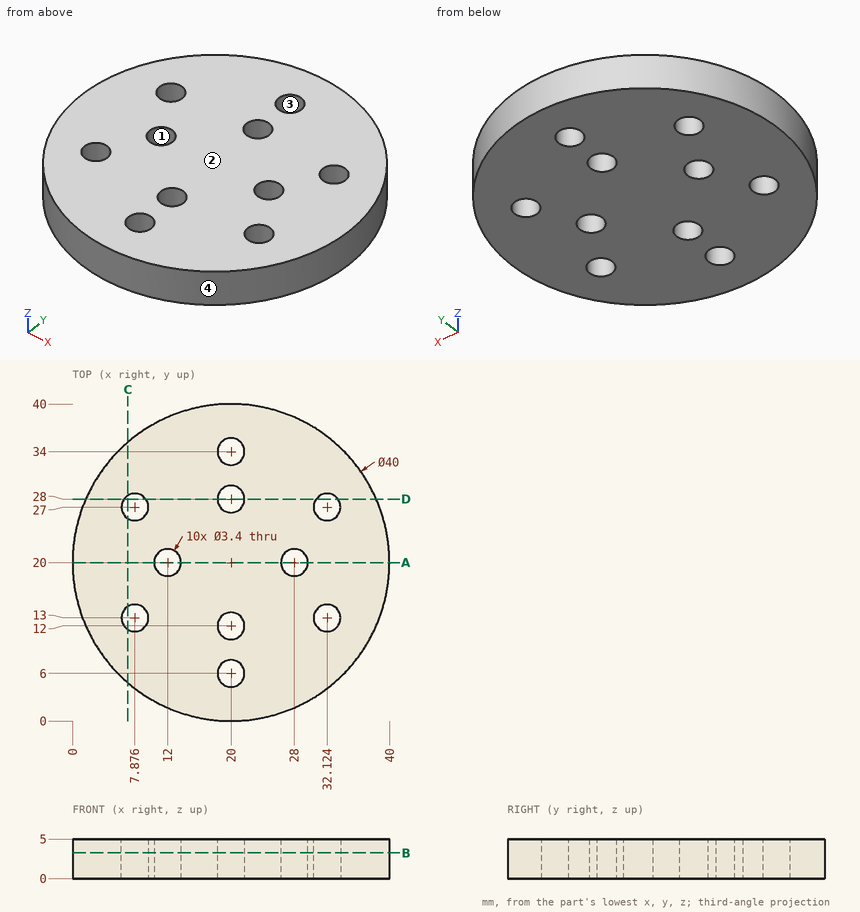
Here's the drawing with two shaded views (mm, measured from the low corner). I have some questions. Give positions to 0.01 mm unless a question says otherwise; leave off trailing zeros. Loops run counter-clockwise (first coordinate to the right, second up) from the corner with the lowest first, then second, coordinate; pieces in that order, holes last. Notation, with made-up numbers: M 1,-22 L 32,-22 A25 cw 32,8 Z; hole C 36,8 d1. An arc over 180 degrees is marked long. One line per item, written item: value.
(1) I need wall thicknesses on line 1 (Y direction, x = 20, z = 2.6); line 2 (X direction, y = 26, z = 1.35); line 3 (Y direction, x = 32, z = 2.95) (1 decimal). Which ranges of each line are inside material? Lowest first, please.
Returned:
line 1: 0 to 4.3, 7.7 to 10.3, 13.7 to 26.3, 29.7 to 32.3, 35.7 to 40
line 2: 0.92 to 6.5, 9.25 to 30.75, 33.5 to 39.08
line 3: 4 to 11.3, 14.7 to 25.3, 28.7 to 36
(2) Suppose I cut it at A-A on y = 20. List the corners of the cut face in (x, z) for me.
Returned:
outline: M 0,0 L 10.3,0 L 10.3,5 L 0,5 Z; M 13.7,0 L 26.3,0 L 26.3,5 L 13.7,5 Z; M 29.7,0 L 40,0 L 40,5 L 29.7,5 Z
(3) We'd pull the mould along X, two halves only. Please class the marked faces 1, 2, 3 and 4: released by +X, released by -X, zero draft, split by the parting line, or undercut.
Returned:
face 1: undercut
face 2: zero draft
face 3: undercut
face 4: split by the parting line
(4) Suppose I cut it at D-D on y = 28. List the corners of the cut face in (x, z) for me.
Returned:
outline: M 1.67,0 L 6.5,0 L 6.5,5 L 1.67,5 Z; M 9.25,0 L 18.3,0 L 18.3,5 L 9.25,5 Z; M 21.7,0 L 30.75,0 L 30.75,5 L 21.7,5 Z; M 33.5,0 L 38.33,0 L 38.33,5 L 33.5,5 Z
(5) Will these pins go through, and if not, where does the flat tip stop? pin 1 (12 mm diameter, centred on x = 23, y = 28.5, fed in from -Z); pin 2 (1 mm diameter, centred on y = 15.5, z = 1.5, fed in from +X).
Returned:
pin 1: z = 0
pin 2: x = 39.6
(6) Suppose I cut it at B-B on z = 3.25. Count the separate pieces of the cut face and the enclosed holes in it, plus the area to 3 significant figures.
Returned:
separate pieces: 1
enclosed holes: 10
area: 1,170 mm^2
(7) Suppose I cut it at C-C on x = 7. List the corners of the cut face in (y, z) for me.
Returned:
outline: M 4.8,0 L 11.54,0 L 11.54,5 L 4.8,5 Z; M 14.46,0 L 25.54,0 L 25.54,5 L 14.46,5 Z; M 28.46,0 L 35.2,0 L 35.2,5 L 28.46,5 Z
